Geometry: final body of the model. Coordinates: model frame, mm. A direction names the side the tool comes from. Give positions to 0.01 mm unless a question says otherwise; leave off trailing zeros. Loops run counter-clockwise (first coordinate to the right, second up) from the corner with the lowest first, then second, coordinate; pieces in that order, holes last. Notation, with made-up numbers: (-34, 24.25) - (-26, 24.25) arc R15 cw to (-26, 51.25) - close; hole circle Ø2 at (55, 32.25). An arc over 180 degrees is marked (long way). Answer in a Markdown table with one row per item.
from build123d import *

# Parameters (mm, degrees)
F1_DEPTH = 26.05
F2_R     = 1.55
F3_DEPTH = 5
F4_R     = 1.55
F5_DEPTH = 3
F6_DEPTH = 2


with BuildPart() as f1:
    # F0 (on Front) → F1 (new body)
    with BuildSketch(Plane.XZ):
        Polygon((0, 90), (0, 0), (25.25, 0), (25.25, 69), (6.25, 69), (6.25, 90), align=None)
    extrude(amount=-F1_DEPTH)

    # F2 (on face) → F3 (cut)
    with BuildSketch(Plane.YZ.offset(25.25)):
        with Locations((9.715, 43.7)):
            Circle(F2_R)
        with Locations((6.59, 25.15)):
            Circle(F2_R)
        with Locations((3.465, 6.6)):
            Circle(F2_R)
    extrude(amount=-F3_DEPTH, mode=Mode.SUBTRACT)

    # F4 (on face) → F5 (cut)
    with BuildSketch(Plane.XY.offset(69)):
        with Locations((21.75, 12.84)):
            Circle(F4_R)
    extrude(amount=-F5_DEPTH, mode=Mode.SUBTRACT)

    # F2 (on face) → F6 (cut)
    with BuildSketch(Plane.YZ.offset(25.25)):
        with Locations((12.84, 65.5)):
            Circle(F2_R)
    extrude(amount=-F6_DEPTH, mode=Mode.SUBTRACT)


solid = f1.part
Q1. First-contact query: pin 1 (1.9 mm diameter, centred on y = 9.715, z = 43.7, fed in from +X); pin 2 (0.9 mm diameter, centred on x = 22, y = 13.5, fed in from +Z); pin 3 (5 mm diameter, centred on y = 5.5, z = 73.5, fed in from +X). Flat tips, straight axial feed; report the tip coordinate or a pass-through.
Check values:
| item | result |
|---|---|
| pin 1 | x = 20.25 |
| pin 2 | z = 66 |
| pin 3 | x = 6.25 |
Q2. Cut plane A-A (y = 6.59). Output: boundary loops of the cut face in (x, z), and give its area (3 significant figures).
Check values:
| item | result |
|---|---|
| outline | (0, 0) - (25.25, 0) - (25.25, 23.6) - (20.25, 23.6) - (20.25, 26.7) - (25.25, 26.7) - (25.25, 69) - (6.25, 69) - (6.25, 90) - (0, 90) - close |
| area | 1,860 mm² |
Q3. Cut plane D-D (z = 6.6). Output: boundary loops of the cut face in (x, y) (3 decimals).
Check values:
| item | result |
|---|---|
| outline | (0, 0) - (25.25, 0) - (25.25, 1.915) - (20.25, 1.915) - (20.25, 5.015) - (25.25, 5.015) - (25.25, 26.05) - (0, 26.05) - close |
Q4. Material intervals for line 1 along Y through (x, z) = (24.2, 65.5); line 2 along X through (y, z) = (12.84, 67.75); line 3 along Z through (x, y) = (21.3, 6.59), sorted ascending.
Check values:
| item | result |
|---|---|
| line 1 | 0 to 11.29, 14.39 to 26.05 |
| line 2 | 0 to 20.2, 23.3 to 25.25 |
| line 3 | 0 to 23.6, 26.7 to 69 |
Q5. Cut plane C-C (x = 16). Output: boundary loops of the cut face in (y, z).
Check values:
| item | result |
|---|---|
| outline | (0, 0) - (26.05, 0) - (26.05, 69) - (0, 69) - close |
Q6. Cut plane B-B (z = 25.15). Output: boundary loops of the cut face in (x, y), and give its area (3 significant figures).
Check values:
| item | result |
|---|---|
| outline | (0, 0) - (25.25, 0) - (25.25, 5.04) - (20.25, 5.04) - (20.25, 8.14) - (25.25, 8.14) - (25.25, 26.05) - (0, 26.05) - close |
| area | 642 mm² |
Q7. Draft query along Y for faces 1 (the flat face through (23.25, 13, 65)), 2 (the cylindrical face through (22.78, 7.42, 26.46)), 3 (the flat face through (0, 13, 46)), 4 (the flat face through (12, 0, 36)). Return one class per face: pulls with the +Y half, pulls with the -Y half, needs draft (parallel to the pull), parting line crosses it, or undercut.
Check values:
| item | result |
|---|---|
| face 1 | undercut |
| face 2 | undercut |
| face 3 | needs draft |
| face 4 | pulls with the -Y half |
Q8. Reachability of faces 5 (the cylindrical face through (22.58, 14.15, 67.52)), 6 (the flat face through (12, 13, 0)), 7 (the flat face through (3, 13, 90)), 8 (the flat face through (6.25, 13, 79)), 9 (the flat face through (20.25, 3, 7)) from +Z, -Z, +X, -X, +Y, -Y: full face, straight path, thin tool, end or side. Return the list, or none.
Check values:
| item | result |
|---|---|
| face 5 | +Z |
| face 6 | -Z, +X, -X, +Y, -Y |
| face 7 | +Z, +X, -X, +Y, -Y |
| face 8 | +Z, +X, +Y, -Y |
| face 9 | +X |
